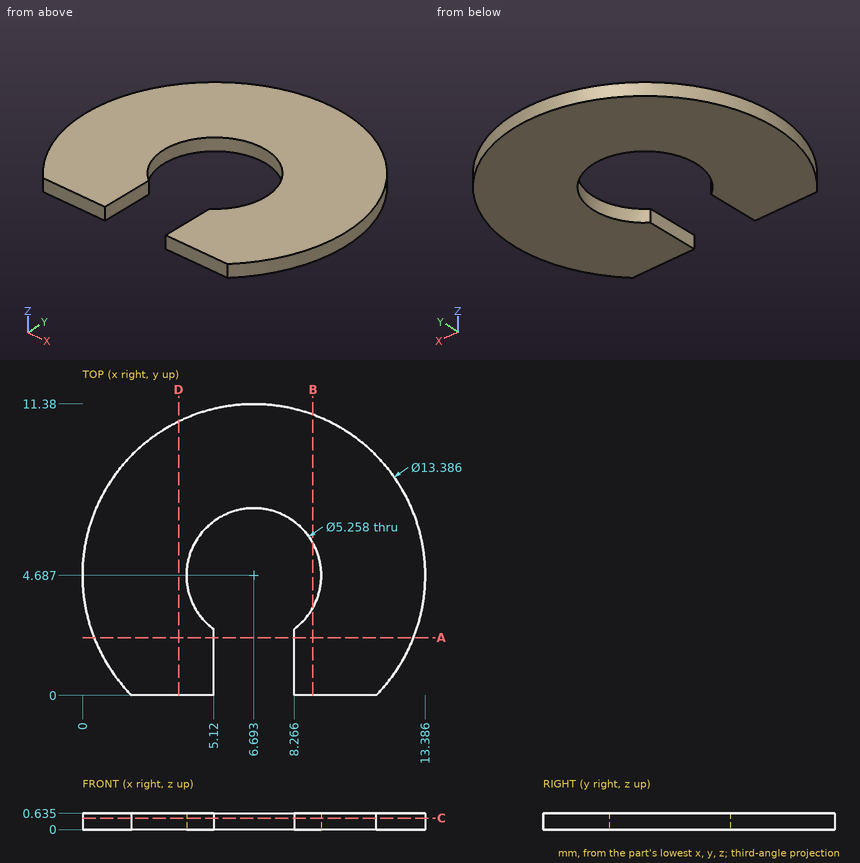
Geometry: see drawing. Coordinates: mm, zero at the bounding-box minimum. Coordinates: 2 decimals unless noted, no trailing zeros. Loops run counter-clockwise (first coordinate to the right, second up) from the corner with the lowest first, then second, coordinate; pieces in that order, holes last. Notation, with made-up numbers: M 9,25.5 L 35,25.5 A29 cw 35,53.5 Z; hole C -29,-9.5 d11. An arc over 180 degrees is marked long. Answer in a Markdown table with one row per item.
Q1. Section D-D on x = 3.75. Return the cut outline in (y, z) (1 decimal).
Answers below:
| item | result |
|---|---|
| outline | M 0,0 L 10.7,0 L 10.7,0.6 L 0,0.6 Z |
Q2. Section C-C on z = 0.45. Return the cut outline in (x, y) (1 decimal).
Answers below:
| item | result |
|---|---|
| outline | M 1.9,0 L 5.1,0 L 5.1,2.6 A2.6 cw long 8.3,2.6 L 8.3,0 L 11.5,0 A6.7 ccw long Z |
Q3. Section B-B on x = 9. Return the cut outline in (y, z) (1 decimal).
Answers below:
| item | result |
|---|---|
| outline | M 0,0 L 3.4,0 L 3.4,0.6 L 0,0.6 Z; M 5.9,0 L 11,0 L 11,0.6 L 5.9,0.6 Z |
Q4. Section A-A on y = 2.25. Return the cut outline in (x, z) (1 decimal).
Answers below:
| item | result |
|---|---|
| outline | M 0.5,0 L 5.1,0 L 5.1,0.6 L 0.5,0.6 Z; M 8.3,0 L 12.9,0 L 12.9,0.6 L 8.3,0.6 Z |
Q5. First-contact query: pin 1 (3 mm diameter, centred on x = 6.69, y = 4.69, fed in from -Z). Flat tip, straight axial feed; report the tip coordinate or a pass-through.
Answers below:
| item | result |
|---|---|
| pin 1 | passes through |
Q6. Ray query, probe 1 along X at (y, z) = (4.5, 0.25) (1 decimal); probe 2 along X at (y, z) = (7, 0.15) (1 decimal); probe 3 along Y at (x, z) = (4.5, 0.3) (1 decimal). Return the intervals inside material, ascending. Write a range as from..to.
Answers below:
| item | result |
|---|---|
| probe 1 | x = 0..4.1, 9.3..13.4 |
| probe 2 | x = 0.4..5.4, 7.9..13 |
| probe 3 | y = 0..3.2, 6.1..11 |
